Could you check a few things on this model? Use its own coordinates, in mm. A direction names the side the tool comes from. Give positions to 0.01 mm unless a question says otherwise; leave off trailing zeros. Loops run counter-clockwise (first coordinate to the right, second up) from the corner with the lowest first, then second, coordinate; pieces in that order, holes last. Notation, with made-up numbers: (60, 48) - (110, 48) arc R33 cw to (110, 85) - close; hole circle Ø11 at (-29, -10.5). An arc over 180 degrees is marked (long way). Use CSV: the item, a comma, the result in double quotes.
Autodesk Inventor part; units mm, degrees
ref_plane "YZ Plane" through (0, 0, 0) normal (1, 0, 0) x (0, 1, 0)
ref_plane "XZ Plane" through (0, 0, 0) normal (0, 1, 0) x (-1, 0, 0)
ref_plane "XY Plane" through (0, 0, 0) normal (0, 0, 1) x (1, 0, 0)
sketch "Эскиз1" plane through (0, 0, 0) normal (1, 0, 0) x (0, 1, 0)
  line L0 (-4.5638, 0) -> (-4.5638, 1)
  line L1 (-4.5638, 1) -> (15.4362, 1)
  line L2 (15.4362, 1) -> (15.4362, -19)
  line L3 (15.4362, -19) -> (14.4362, -19)
  line L4 (14.4362, -19) -> (14.4362, 0)
  line L5 (14.4362, 0) -> (-4.5638, 0)
  point P0 (0, 0)
  dimension "d0" = 1
  dimension "d1" = 20
  dimension "d2" = 20
  dimension "d3" = 1
  dimension "d4" = 19
extrude "Выдавливание1" add sketch "Эскиз1" along normal blind 580
properties part number "уголок 580" material "Алюминий 6061"
1) Which directions (+Z, -Z, +X, -X, +Y, -Y) give clear straight access to the entire face, cutting with the end or side of a thin tool? Please do faces 1 (the flat face through (286, 14.436, -10)), 2 (the flat face through (286, 15.436, -9)).
Answer below:
face 1,"-Z, +X, -X, -Y"
face 2,"+Z, -Z, +X, -X, +Y"
2) Suppose I cut it at C-C (y = 10.5). Please give me the cut outline in (x, z), plus the area to 3 significant figures.
Answer below:
outline,"(0, 0) - (580, 0) - (580, 1) - (0, 1) - close"
area,"580 mm2"
3) I need wall thicknesses on line 1 along Y through (x, z) = (353, -17); line 2 along Z through (x, y) = (373.5, 4.5). Which ranges of each line are inside material? Lowest first, please.
Answer below:
line 1,"y = 14.44 to 15.44"
line 2,"z = 0 to 1"
4) Suppose I cut it at A-A (x = 279.5). Please give me the cut outline in (y, z), plus the area to 3 significant figures.
Answer below:
outline,"(-4.56, 0) - (14.44, 0) - (14.44, -19) - (15.44, -19) - (15.44, 1) - (-4.56, 1) - close"
area,"39.0 mm2"
5) I'm going to push flat-ended pins straight in: P1, Ø9.5, axis at x = 409.5, z = -6, coming from the -Y side; P2, Ø8, axis at y = 11, z = -13.5, coming from the -X side; P3, Ø5, axis at y = 11.5, z = -4, coming from the -X side; P4, Ø2, axis at x = 496.5, y = 0.5, coming from the -Z side. Where does each tip first touch, or does it pass through?
Answer below:
P1,"stops at y = 14.44"
P2,"stops at x = 0"
P3,"passes through"
P4,"stops at z = 0"
6) Suppose I cut it at B-B (z = -14.5). Please give me the cut outline in (x, y), plus the area to 3 significant figures.
Answer below:
outline,"(0, 14.44) - (580, 14.44) - (580, 15.44) - (0, 15.44) - close"
area,"580 mm2"
